Design review of the part built by this model. Coordinates are the model's own, in mm. A direction names the side the tool comes from. Round coordinates to 2 decimals unless told otherwise and drop trailing zeros. Order: outer loops, then holes, each group sorted by start corner. A loop starts at its lowest first (then second) coordinate and runs counter-clockwise, first axis right, second up. Notation, with made-up numbers: (-21, 66.25) - (0, 66.25) arc R11 ccw to (0, 77.25) - close; hole circle Ø9 at (66.5, 37). An arc over 180 degrees is marked (long way). Use CSV: the item, a comma, the result in double quotes.
from build123d import *

# Parameters (mm, degrees)
BOSS_EXTRUDE1_DEPTH           = 4.4
CUT_EXTRUDE1_DEPTH            = 2
BOSS_EXTRUDE3_START           = 1.2
BOSS_EXTRUDE3_DEPTH           = 1.2
CSK_FOR_M3_SFHCS1_D           = 3.4
CSK_FOR_M3_SFHCS1_CSINK_D     = 6.72
CSK_FOR_M3_SFHCS1_CSINK_ANGLE = 90
CUT_EXTRUDE2_DEPTH            = 112.396790798
F_4_0_4_DIAMETER_HOLE1_D      = 4


with BuildPart() as part:
    # Sketch1 → Boss-Extrude1 (new body)
    with BuildSketch(Plane(origin=(0, 0, 0), x_dir=(1, 0, 0), z_dir=(0, 1, 0))):
        with BuildLine():
            Line((-89.85, 59.75), (89.85, 59.75))
            ThreePointArc((89.85, 59.75), (92.678427125, 58.578427125), (93.85, 55.75))
            Line((93.85, 55.75), (93.85, -55.75))
            ThreePointArc((93.85, -55.75), (92.678427125, -58.578427125), (89.85, -59.75))
            Line((89.85, -59.75), (-89.85, -59.75))
            ThreePointArc((-89.85, -59.75), (-92.678427125, -58.578427125), (-93.85, -55.75))
            Line((-93.85, -55.75), (-93.85, 55.75))
            ThreePointArc((-93.85, 55.75), (-92.678427125, 58.578427125), (-89.85, 59.75))
        make_face()
    extrude(amount=BOSS_EXTRUDE1_DEPTH)

    # Sketch2 → Cut-Extrude1 (cut)
    with BuildSketch(Plane(origin=(0, 4.4, 0), x_dir=(1, 0, 0), z_dir=(0, 1, 0))):
        with BuildLine():
            Line((-83.340524981, -53.55), (-5.809475019, -53.55))
            ThreePointArc((-5.809475019, -53.55), (0, -49.05), (5.809475019, -53.55))
            Line((5.809475019, -53.55), (83.340524981, -53.55))
            ThreePointArc((83.340524981, -53.55), (84.690787612, -51.035597818), (87.05, -49.429501801))
            Line((87.05, -49.429501801), (87.05, 49.429501801))
            ThreePointArc((87.05, 49.429501801), (84.690787612, 51.035597818), (83.340524981, 53.55))
            Line((83.340524981, 53.55), (5.809475019, 53.55))
            ThreePointArc((5.809475019, 53.55), (0, 49.05), (-5.809475019, 53.55))
            Line((-5.809475019, 53.55), (-83.340524981, 53.55))
            ThreePointArc((-83.340524981, 53.55), (-84.690787612, 51.035597818), (-87.05, 49.429501801))
            Line((-87.05, 49.429501801), (-87.05, -49.429501801))
            ThreePointArc((-87.05, -49.429501801), (-84.690787612, -51.035597818), (-83.340524981, -53.55))
        make_face()
    extrude(amount=-CUT_EXTRUDE1_DEPTH, mode=Mode.SUBTRACT)

    # Sketch3 → Boss-Extrude3 (add)
    with BuildSketch(Plane(origin=(0, 4.4, 0), x_dir=(1, 0, 0), z_dir=(0, 1, 0)).offset(BOSS_EXTRUDE3_START)):
        with BuildLine():
            Line((-88.8, 50.814436283), (-88.8, -50.814436283))
            ThreePointArc((-88.8, -50.814436283), (-85.940146797, -52.264440377), (-84.907359313, -55.3))
            Line((-84.907359313, -55.3), (-4.242640687, -55.3))
            ThreePointArc((-4.242640687, -55.3), (0, -50.8), (4.242640687, -55.3))
            Line((4.242640687, -55.3), (84.907359313, -55.3))
            ThreePointArc((84.907359313, -55.3), (85.940146797, -52.264440377), (88.8, -50.814436283))
            Line((88.8, -50.814436283), (88.8, 50.814436283))
            ThreePointArc((88.8, 50.814436283), (85.940146797, 52.264440377), (84.907359313, 55.3))
            Line((84.907359313, 55.3), (4.242640687, 55.3))
            ThreePointArc((4.242640687, 55.3), (0, 50.8), (-4.242640687, 55.3))
            Line((-4.242640687, 55.3), (-84.907359313, 55.3))
            ThreePointArc((-84.907359313, 55.3), (-85.940146797, 52.264440377), (-88.8, 50.814436283))
        make_face()
        with BuildLine():
            Line((-87.05, 49.429501801), (-87.05, -49.429501801))
            ThreePointArc((-87.05, -49.429501801), (-84.690787612, -51.035597818), (-83.340524981, -53.55))
            Line((-83.340524981, -53.55), (-5.809475019, -53.55))
            ThreePointArc((-5.809475019, -53.55), (0, -49.05), (5.809475019, -53.55))
            Line((5.809475019, -53.55), (83.340524981, -53.55))
            ThreePointArc((83.340524981, -53.55), (84.690787612, -51.035597818), (87.05, -49.429501801))
            Line((87.05, -49.429501801), (87.05, 49.429501801))
            ThreePointArc((87.05, 49.429501801), (84.690787612, 51.035597818), (83.340524981, 53.55))
            Line((83.340524981, 53.55), (5.809475019, 53.55))
            ThreePointArc((5.809475019, 53.55), (0, 49.05), (-5.809475019, 53.55))
            Line((-5.809475019, 53.55), (-83.340524981, 53.55))
            ThreePointArc((-83.340524981, 53.55), (-84.690787612, 51.035597818), (-87.05, 49.429501801))
        make_face(mode=Mode.SUBTRACT)
    extrude(amount=-BOSS_EXTRUDE3_DEPTH)

    # CSK for M3 SFHCS1 (through all)
    with Locations(Plane(origin=(-54.95207322, 0, 58.575897403), x_dir=(1, 0, 0), z_dir=(0, -1, 0))):
        with Locations((-34.19792678, -113.625897403), (-34.19792678, -3.525897403), (144.10207322, -3.525897403), (144.10207322, -113.625897403), (54.95207322, -3.525897403), (54.95207322, -113.625897403)):
            CounterSinkHole(CSK_FOR_M3_SFHCS1_D / 2, CSK_FOR_M3_SFHCS1_CSINK_D / 2, counter_sink_angle=CSK_FOR_M3_SFHCS1_CSINK_ANGLE)

    # Sketch8 → Cut-Extrude2 (cut, through all)
    with BuildSketch(Plane.XZ):
        with BuildLine():
            Line((-0.65, -16.75), (74.35, -16.75))
            ThreePointArc((74.35, -16.75), (80.35, -22.75), (74.35, -28.75))
            Line((74.35, -28.75), (-0.65, -28.75))
            ThreePointArc((-0.65, -28.75), (-6.65, -22.75), (-0.65, -16.75))
        make_face()
        with BuildLine():
            Line((-50.65, 28.75), (74.35, 28.75))
            ThreePointArc((74.35, 28.75), (80.35, 22.75), (74.35, 16.75))
            Line((74.35, 16.75), (-50.65, 16.75))
            ThreePointArc((-50.65, 16.75), (-56.65, 22.75), (-50.65, 28.75))
        make_face()
    extrude(amount=-CUT_EXTRUDE2_DEPTH, mode=Mode.SUBTRACT)

    # Ø4.0 (4) Diameter Hole1 (through all)
    with Locations(Plane(origin=(0, 0, 0), x_dir=(-1, 0, 0), z_dir=(0, -1, 0))):
        with Locations((75.65, -35.25), (75.65, 33.75), (-76.35, 33.75), (-76.35, -35.25)):
            Hole(F_4_0_4_DIAMETER_HOLE1_D / 2)


solid = part.part
1) We need section C-C (y = 3.45). Give the boundary of the cut face in (x, z), then the cut area to 3 significant figures.
Data:
outline,"(-93.85, -55.75) arc R4 ccw to (-89.85, -59.75) - (89.85, -59.75) arc R4 ccw to (93.85, -55.75) - (93.85, 55.75) arc R4 ccw to (89.85, 59.75) - (-89.85, 59.75) arc R4 ccw to (-93.85, 55.75) - close; hole circle Ø3.4 at (-89.15, -55.05); hole circle Ø3.4 at (-89.15, 55.05); hole (-87.05, -49.43) arc R6 cw to (-83.34, -53.55) - (-5.81, -53.55) arc R6 cw to (5.81, -53.55) - (83.34, -53.55) arc R6 cw to (87.05, -49.43) - (87.05, 49.43) arc R6 cw to (83.34, 53.55) - (5.81, 53.55) arc R6 cw to (-5.81, 53.55) - (-83.34, 53.55) arc R6 cw to (-87.05, 49.43) - close; hole circle Ø3.4 at (0, -55.05); hole circle Ø3.4 at (0, 55.05); hole circle Ø3.4 at (89.15, -55.05); hole circle Ø3.4 at (89.15, 55.05)"
area,"3,830 mm2"
2) Insertion check: pin 1 Ø5 at (x, z) = (-29, 17.5) entering from +Y; pin 2 Ø1 at (y, z) = (5, 23) entering from +X; pin 3 Ø1 at (x, y) = (27, 5) entering from +Z. Each pin has a flat end and moves straight along its axis. Give the tip position at first contact, or say it passes through.
Data:
pin 1,"stops at y = 2.4"
pin 2,"stops at x = 88.8"
pin 3,"stops at z = 55.3"
3) The part is to be moulded in two halves that separate along Z. For faces 1 (the face through (1, 0, -1)), 2 (the face through (92.709, 2.169, 58.547)), 3 (the face through (0.11, 4.02, -49.05)), say which applies: +Z half, -Z half, draft (parallel to the pull), parting line (faces both ways), or undercut.
Data:
face 1,"draft"
face 2,"+Z half"
face 3,"undercut"
4) To check wall thickness, follow L1, parallel to Z at x = 23.5, y = 1.75; L2, parallel to X at y = 3.35, z = 55.05; L3, parallel to X at y = 1.35, z = -33.75. State the ranges of each line that lie inside material, in increasing order. Write a range as from..to.
Data:
L1,"z = -59.75..-28.75, -16.75..16.75, 28.75..59.75"
L2,"x = -93.85..-90.85, -87.45..-1.7, 1.7..87.45, 90.85..93.85"
L3,"x = -93.85..-77.65, -73.65..74.35, 78.35..93.85"
5) We need section A-A (z = 22.75). Give the boundary of the cut face in (x, y), then the cut area to 3 significant figures.
Data:
outline,"(-93.85, 0) - (-56.65, 0) - (-56.65, 2.4) - (-87.05, 2.4) - (-87.05, 5.6) - (-88.8, 5.6) - (-88.8, 4.4) - (-93.85, 4.4) - close; (80.35, 0) - (93.85, 0) - (93.85, 4.4) - (88.8, 4.4) - (88.8, 5.6) - (87.05, 5.6) - (87.05, 2.4) - (80.35, 2.4) - close"
area,"153 mm2"
6) For faces 4 (the face through (-0.11, 4.02, 49.05)), 5 (the face through (80.35, 1.18, 22.88)), 6 (the face through (-1, 2, -59.75)), list the 3-axis set-ups (+Z, -Z, +X, -X, +Y, -Y) from which the entire face can be reached by the end or side of a thin tool; tool diameter is ignored.
Data:
face 4,"+Y"
face 5,"+Y, -Y"
face 6,"-Z, +X, -X, +Y, -Y"
7) We need section B-B (x = 32). Give the boundary of the cut face in (y, z), then the cut area to 3 significant figures.
Data:
outline,"(0, -59.75) - (4.4, -59.75) - (4.4, -55.3) - (5.6, -55.3) - (5.6, -53.55) - (2.4, -53.55) - (2.4, -28.75) - (0, -28.75) - close; (0, -16.75) - (2.4, -16.75) - (2.4, 16.75) - (0, 16.75) - close; (0, 28.75) - (2.4, 28.75) - (2.4, 53.55) - (5.6, 53.55) - (5.6, 55.3) - (4.4, 55.3) - (4.4, 59.75) - (0, 59.75) - close"
area,"258 mm2"
8) We need section D-D (x = -17.5). Give the boundary of the cut face in (y, z), then the cut area to 3 significant figures.
Data:
outline,"(0, -59.75) - (4.4, -59.75) - (4.4, -55.3) - (5.6, -55.3) - (5.6, -53.55) - (2.4, -53.55) - (2.4, 16.75) - (0, 16.75) - close; (0, 28.75) - (2.4, 28.75) - (2.4, 53.55) - (5.6, 53.55) - (5.6, 55.3) - (4.4, 55.3) - (4.4, 59.75) - (0, 59.75) - close"
area,"287 mm2"
